```python
from build123d import *

# Parameters (mm, degrees)
SKETCH1_R           = 38.1
BOSS_EXTRUDE1_DEPTH = 6.35
SKETCH2_R           = 6.35
BOSS_EXTRUDE2_DEPTH = 12.7
SKETCH3_R           = 6.35
BOSS_EXTRUDE3_DEPTH = 12.7
SKETCH4_R           = 3.175
CUT_EXTRUDE1_DEPTH  = 3.175


with BuildPart() as part:
    # Sketch1 → Boss-Extrude1 (new body)
    with BuildSketch(Plane.XY):
        Circle(SKETCH1_R)
    extrude(amount=BOSS_EXTRUDE1_DEPTH)

    # Sketch2 → Boss-Extrude2 (add)
    with BuildSketch(Plane.XY.offset(6.35)):
        Circle(SKETCH2_R)
    extrude(amount=BOSS_EXTRUDE2_DEPTH)

    # Sketch3 → Boss-Extrude3 (add)
    with BuildSketch(Plane.XY.offset(19.05)):
        with Locations(Location((0, -1.905, 0), (0, 0, 171.373073441))):
            Circle(SKETCH3_R)
    extrude(amount=BOSS_EXTRUDE3_DEPTH)

    # Sketch4 → Cut-Extrude1 (cut)
    with BuildSketch(Plane(origin=(0, 0, 0), x_dir=(-1, 0, 0), z_dir=(0, 0, -1))):
        with Locations((-25.4, 0)):
            Circle(SKETCH4_R)
        with Locations((-12.7, 21.997045256)):
            Circle(SKETCH4_R)
        with Locations((12.7, 21.997045256)):
            Circle(SKETCH4_R)
        with Locations((25.4, 0)):
            Circle(SKETCH4_R)
        with Locations((12.7, -21.997045256)):
            Circle(SKETCH4_R)
        with Locations((-12.7, -21.997045256)):
            Circle(SKETCH4_R)
    extrude(amount=-CUT_EXTRUDE1_DEPTH, mode=Mode.SUBTRACT)


solid = part.part
```
Build history of the part. All positions in model axes, mm. A direction names the side the tool comes from. Round coordinates to 2 decimals unless told otherwise and drop trailing zeros. Order: outer loops, then holes, each group sorted by start corner. A loop starts at its lowest first (then second) coordinate and runs counter-clockwise, first axis right, second up. Notation, with made-up numbers: (52.25, -27.75) - (66.25, -27.75) arc R25 ccw to (66.25, -13.75) - close; hole circle Ø3 at (83, 73). An arc over 180 degrees is marked (long way). Use a Markdown table: item, result.
1) Saw through at B-B on z = 5. Write the cut outline in (x, y), and give its area (3 significant figures).
Recorded:
| item | result |
|---|---|
| outline | circle Ø76.2 at (0, 0) |
| area | 4,560 mm² |
2) Tool access for faces 1 (the face through (0, -7, 19.05)), 2 (the face through (25, 0, 3.175)), 3 (the face through (-6.274, -2.882, 25.311)): list every direction of +Z, -Z, +X, -X, +Y, -Y with a clear straight run to the whole face (end or side of a thin tool).
Recorded:
| item | result |
|---|---|
| face 1 | -Y |
| face 2 | -Z |
| face 3 | +Z |
3) Flat gauge pins, fed straight in: pin 1 Ø5 at (x, y) = (12.7, -22) entering from -Z (3 decimals); pin 2 Ø5.5 at (x, y) = (-12.7, 22) entering from +Z; pin 3 Ø10 at (y, z) = (14.5, 22.5) entering from +X. Where does each tip first touch, or does it go through?
Recorded:
| item | result |
|---|---|
| pin 1 | stops at z = 3.175 |
| pin 2 | stops at z = 6.35 |
| pin 3 | passes through |
4) Wall check: L1, parallel to Y at x = 12.7, z = 0.95; L2, parallel to Z at x = -28, y = 20.5; L3, parallel to Y at x = 12, z = 2. Give the ranges that are in metal, low to high.
Recorded:
| item | result |
|---|---|
| L1 | y = -35.92 to -25.17, -18.82 to 18.82, 25.17 to 35.92 |
| L2 | z = 0 to 6.35 |
| L3 | y = -36.16 to -25.09, -18.9 to 18.9, 25.09 to 36.16 |
5) Pull direction Y, two halves, no side cores. Call faces 4 (the face through (-1.38, -6.2, 12.61)), 5 (the face through (-1, 5, 19.05)), 6 (the face through (-28.43, 0.95, 1.57)): pulls with the +Y half, pulls with the -Y half, needs draft (parallel to the pull), parting line crosses it, or undercut.
Recorded:
| item | result |
|---|---|
| face 4 | parting line crosses it |
| face 5 | needs draft |
| face 6 | undercut |
6) Saw through at A-A on x = 0. Write the cut outline in (y, z) (3 decimals).
Recorded:
| item | result |
|---|---|
| outline | (-38.1, 0) - (38.1, 0) - (38.1, 6.35) - (6.35, 6.35) - (6.35, 19.05) - (4.445, 19.05) - (4.445, 31.75) - (-8.255, 31.75) - (-8.255, 19.05) - (-6.35, 19.05) - (-6.35, 6.35) - (-38.1, 6.35) - close |
7) Saw through at D-D on y = -16. Write the cut outline in (x, z), and give its area (3 significant figures).
Recorded:
| item | result |
|---|---|
| outline | (-34.58, 0) - (34.58, 0) - (34.58, 6.35) - (-34.58, 6.35) - close |
| area | 439 mm² |
8) Saw through at C-C on x = -25. Write the cut outline in (y, z) (3 decimals), and give its area (3 significant figures).
Recorded:
| item | result |
|---|---|
| outline | (-28.751, 0) - (-3.15, 0) - (-3.15, 3.175) - (3.15, 3.175) - (3.15, 0) - (28.751, 0) - (28.751, 6.35) - (-28.751, 6.35) - close |
| area | 345 mm² |
